```python
from build123d import *

# Parameters (mm, degrees)
SKETCH1_W               = 28.9
SKETCH1_H               = 5.8
BOSS_EXTRUDE1_DEPTH     = 2.5
CUT_EXTRUDE1_DEPTH      = 15.948662147
CUT_EXTRUDE1_DEPTH_BACK = 15.948662147
SKETCH2_R               = 0.525
FILL_START              = -2.5
FILL_PATTERN1_OUTLINE_R = 0.525
FILL_PATTERN1_DEPTH     = 5
SKETCH4_W               = 28.9
SKETCH4_H               = 0.2
BOSS_EXTRUDE2_DEPTH     = 2.5


# Read off the part's stored shape, not the designer's step: Fill Pattern1
with BuildPart() as part:
    # Sketch1 → Boss-Extrude1 (new, symmetric)
    with BuildSketch(Plane.XY):
        Rectangle(SKETCH1_W, SKETCH1_H)
    extrude(amount=BOSS_EXTRUDE1_DEPTH, both=True)

    # Sketch2 → Cut-Extrude1 (cut, two sides: drawn at the far end of the back side and taken through both)
    with BuildSketch(Plane.XY.offset(-CUT_EXTRUDE1_DEPTH_BACK)):
        Circle(SKETCH2_R)
    extrude(amount=CUT_EXTRUDE1_DEPTH + CUT_EXTRUDE1_DEPTH_BACK, mode=Mode.SUBTRACT)

    # Fill Pattern1 outline → Fill Pattern1 (cut)
    with BuildSketch(Plane.XY.offset(FILL_START)):
        with Locations((13.65, -1.125833025)):
            Circle(FILL_PATTERN1_OUTLINE_R)
        with Locations((-9.75, -1.125833025)):
            Circle(FILL_PATTERN1_OUTLINE_R)
        with Locations((-9.1, 0)):
            Circle(FILL_PATTERN1_OUTLINE_R)
        with Locations((-8.45, 1.125833025)):
            Circle(FILL_PATTERN1_OUTLINE_R)
        with Locations((-7.8, 2.25166605)):
            Circle(FILL_PATTERN1_OUTLINE_R)
        with Locations((-9.1, -2.25166605)):
            Circle(FILL_PATTERN1_OUTLINE_R)
        with Locations((-8.45, -1.125833025)):
            Circle(FILL_PATTERN1_OUTLINE_R)
        with Locations((-7.8, 0)):
            Circle(FILL_PATTERN1_OUTLINE_R)
        with Locations((-7.15, 1.125833025)):
            Circle(FILL_PATTERN1_OUTLINE_R)
        with Locations((-11.05, 1.125833025)):
            Circle(FILL_PATTERN1_OUTLINE_R)
        with Locations((-10.4, 2.25166605)):
            Circle(FILL_PATTERN1_OUTLINE_R)
        with Locations((-11.7, -2.25166605)):
            Circle(FILL_PATTERN1_OUTLINE_R)
        with Locations((-11.05, -1.125833025)):
            Circle(FILL_PATTERN1_OUTLINE_R)
        with Locations((-10.4, -2.25166605)):
            Circle(FILL_PATTERN1_OUTLINE_R)
        with Locations((-9.1, 2.25166605)):
            Circle(FILL_PATTERN1_OUTLINE_R)
        with Locations((-9.75, 1.125833025)):
            Circle(FILL_PATTERN1_OUTLINE_R)
        with Locations((-10.4, 0)):
            Circle(FILL_PATTERN1_OUTLINE_R)
        with Locations((-5.2, -2.25166605)):
            Circle(FILL_PATTERN1_OUTLINE_R)
        with Locations((-3.9, 2.25166605)):
            Circle(FILL_PATTERN1_OUTLINE_R)
        with Locations((-4.55, 1.125833025)):
            Circle(FILL_PATTERN1_OUTLINE_R)
        with Locations((-5.2, 0)):
            Circle(FILL_PATTERN1_OUTLINE_R)
        with Locations((-4.55, -1.125833025)):
            Circle(FILL_PATTERN1_OUTLINE_R)
        with Locations((-3.9, 0)):
            Circle(FILL_PATTERN1_OUTLINE_R)
        with Locations((-3.25, 1.125833025)):
            Circle(FILL_PATTERN1_OUTLINE_R)
        with Locations((-2.6, 2.25166605)):
            Circle(FILL_PATTERN1_OUTLINE_R)
        with Locations((-6.5, 0)):
            Circle(FILL_PATTERN1_OUTLINE_R)
        with Locations((-7.15, -1.125833025)):
            Circle(FILL_PATTERN1_OUTLINE_R)
        with Locations((-7.8, -2.25166605)):
            Circle(FILL_PATTERN1_OUTLINE_R)
        with Locations((-6.5, 2.25166605)):
            Circle(FILL_PATTERN1_OUTLINE_R)
        with Locations((-5.85, 1.125833025)):
            Circle(FILL_PATTERN1_OUTLINE_R)
        with Locations((-5.2, 2.25166605)):
            Circle(FILL_PATTERN1_OUTLINE_R)
        with Locations((-6.5, -2.25166605)):
            Circle(FILL_PATTERN1_OUTLINE_R)
        with Locations((-5.85, -1.125833025)):
            Circle(FILL_PATTERN1_OUTLINE_R)
        with Locations((-13.65, 1.125833025)):
            Circle(FILL_PATTERN1_OUTLINE_R)
        with Locations((-11.7, 2.25166605)):
            Circle(FILL_PATTERN1_OUTLINE_R)
        with Locations((-13, -2.25166605)):
            Circle(FILL_PATTERN1_OUTLINE_R)
        with Locations((-12.35, -1.125833025)):
            Circle(FILL_PATTERN1_OUTLINE_R)
        with Locations((-11.7, 0)):
            Circle(FILL_PATTERN1_OUTLINE_R)
        with Locations((-13, 2.25166605)):
            Circle(FILL_PATTERN1_OUTLINE_R)
        with Locations((-13.65, -1.125833025)):
            Circle(FILL_PATTERN1_OUTLINE_R)
        with Locations((-13, 0)):
            Circle(FILL_PATTERN1_OUTLINE_R)
        with Locations((-12.35, 1.125833025)):
            Circle(FILL_PATTERN1_OUTLINE_R)
        with Locations((7.15, -1.125833025)):
            Circle(FILL_PATTERN1_OUTLINE_R)
        with Locations((7.8, 0)):
            Circle(FILL_PATTERN1_OUTLINE_R)
        with Locations((8.45, 1.125833025)):
            Circle(FILL_PATTERN1_OUTLINE_R)
        with Locations((9.1, 2.25166605)):
            Circle(FILL_PATTERN1_OUTLINE_R)
        with Locations((7.8, -2.25166605)):
            Circle(FILL_PATTERN1_OUTLINE_R)
        with Locations((8.45, -1.125833025)):
            Circle(FILL_PATTERN1_OUTLINE_R)
        with Locations((9.1, 0)):
            Circle(FILL_PATTERN1_OUTLINE_R)
        with Locations((9.75, 1.125833025)):
            Circle(FILL_PATTERN1_OUTLINE_R)
        with Locations((5.85, 1.125833025)):
            Circle(FILL_PATTERN1_OUTLINE_R)
        with Locations((6.5, 2.25166605)):
            Circle(FILL_PATTERN1_OUTLINE_R)
        with Locations((5.2, -2.25166605)):
            Circle(FILL_PATTERN1_OUTLINE_R)
        with Locations((5.85, -1.125833025)):
            Circle(FILL_PATTERN1_OUTLINE_R)
        with Locations((6.5, -2.25166605)):
            Circle(FILL_PATTERN1_OUTLINE_R)
        with Locations((7.8, 2.25166605)):
            Circle(FILL_PATTERN1_OUTLINE_R)
        with Locations((7.15, 1.125833025)):
            Circle(FILL_PATTERN1_OUTLINE_R)
        with Locations((6.5, 0)):
            Circle(FILL_PATTERN1_OUTLINE_R)
        with Locations((11.7, -2.25166605)):
            Circle(FILL_PATTERN1_OUTLINE_R)
        with Locations((13, 2.25166605)):
            Circle(FILL_PATTERN1_OUTLINE_R)
        with Locations((12.35, 1.125833025)):
            Circle(FILL_PATTERN1_OUTLINE_R)
        with Locations((11.7, 0)):
            Circle(FILL_PATTERN1_OUTLINE_R)
        with Locations((13, -2.25166605)):
            Circle(FILL_PATTERN1_OUTLINE_R)
        with Locations((13.65, 1.125833025)):
            Circle(FILL_PATTERN1_OUTLINE_R)
        with Locations((13, 0)):
            Circle(FILL_PATTERN1_OUTLINE_R)
        with Locations((12.35, -1.125833025)):
            Circle(FILL_PATTERN1_OUTLINE_R)
        with Locations((10.4, 0)):
            Circle(FILL_PATTERN1_OUTLINE_R)
        with Locations((9.75, -1.125833025)):
            Circle(FILL_PATTERN1_OUTLINE_R)
        with Locations((9.1, -2.25166605)):
            Circle(FILL_PATTERN1_OUTLINE_R)
        with Locations((10.4, 2.25166605)):
            Circle(FILL_PATTERN1_OUTLINE_R)
        with Locations((11.05, 1.125833025)):
            Circle(FILL_PATTERN1_OUTLINE_R)
        with Locations((11.7, 2.25166605)):
            Circle(FILL_PATTERN1_OUTLINE_R)
        with Locations((10.4, -2.25166605)):
            Circle(FILL_PATTERN1_OUTLINE_R)
        with Locations((11.05, -1.125833025)):
            Circle(FILL_PATTERN1_OUTLINE_R)
        with Locations((-0.65, 1.125833025)):
            Circle(FILL_PATTERN1_OUTLINE_R)
        with Locations((0, 2.25166605)):
            Circle(FILL_PATTERN1_OUTLINE_R)
        with Locations((-1.3, -2.25166605)):
            Circle(FILL_PATTERN1_OUTLINE_R)
        with Locations((-0.65, -1.125833025)):
            Circle(FILL_PATTERN1_OUTLINE_R)
        with Locations((0.65, 1.125833025)):
            Circle(FILL_PATTERN1_OUTLINE_R)
        with Locations((1.3, 2.25166605)):
            Circle(FILL_PATTERN1_OUTLINE_R)
        with Locations((0, -2.25166605)):
            Circle(FILL_PATTERN1_OUTLINE_R)
        with Locations((0.65, -1.125833025)):
            Circle(FILL_PATTERN1_OUTLINE_R)
        with Locations((-3.9, -2.25166605)):
            Circle(FILL_PATTERN1_OUTLINE_R)
        with Locations((-3.25, -1.125833025)):
            Circle(FILL_PATTERN1_OUTLINE_R)
        with Locations((-2.6, 0)):
            Circle(FILL_PATTERN1_OUTLINE_R)
        with Locations((-1.95, 1.125833025)):
            Circle(FILL_PATTERN1_OUTLINE_R)
        with Locations((-1.3, 0)):
            Circle(FILL_PATTERN1_OUTLINE_R)
        with Locations((-1.95, -1.125833025)):
            Circle(FILL_PATTERN1_OUTLINE_R)
        with Locations((-2.6, -2.25166605)):
            Circle(FILL_PATTERN1_OUTLINE_R)
        with Locations((-1.3, 2.25166605)):
            Circle(FILL_PATTERN1_OUTLINE_R)
        with Locations((2.6, -2.25166605)):
            Circle(FILL_PATTERN1_OUTLINE_R)
        with Locations((3.25, -1.125833025)):
            Circle(FILL_PATTERN1_OUTLINE_R)
        with Locations((3.9, 0)):
            Circle(FILL_PATTERN1_OUTLINE_R)
        with Locations((4.55, 1.125833025)):
            Circle(FILL_PATTERN1_OUTLINE_R)
        with Locations((5.2, 0)):
            Circle(FILL_PATTERN1_OUTLINE_R)
        with Locations((4.55, -1.125833025)):
            Circle(FILL_PATTERN1_OUTLINE_R)
        with Locations((3.9, -2.25166605)):
            Circle(FILL_PATTERN1_OUTLINE_R)
        with Locations((5.2, 2.25166605)):
            Circle(FILL_PATTERN1_OUTLINE_R)
        with Locations((1.3, -2.25166605)):
            Circle(FILL_PATTERN1_OUTLINE_R)
        with Locations((2.6, 2.25166605)):
            Circle(FILL_PATTERN1_OUTLINE_R)
        with Locations((1.95, 1.125833025)):
            Circle(FILL_PATTERN1_OUTLINE_R)
        with Locations((1.3, 0)):
            Circle(FILL_PATTERN1_OUTLINE_R)
        with Locations((1.95, -1.125833025)):
            Circle(FILL_PATTERN1_OUTLINE_R)
        with Locations((2.6, 0)):
            Circle(FILL_PATTERN1_OUTLINE_R)
        with Locations((3.25, 1.125833025)):
            Circle(FILL_PATTERN1_OUTLINE_R)
        with Locations((3.9, 2.25166605)):
            Circle(FILL_PATTERN1_OUTLINE_R)
    extrude(amount=FILL_PATTERN1_DEPTH, mode=Mode.SUBTRACT)

    # Sketch4 → Boss-Extrude2 (add, symmetric)
    with BuildSketch(Plane.XY):
        with Locations((0, 3)):
            Rectangle(SKETCH4_W, SKETCH4_H)
        with Locations((0, -3)):
            Rectangle(SKETCH4_W, SKETCH4_H)
    extrude(amount=BOSS_EXTRUDE2_DEPTH, both=True)


solid = part.part
```
Part model, mm, in its own coordinate system. Round coordinates to 2 decimals unless told otherwise and drop trailing zeros. Answer in a Markdown table with one row per item. Add a question column.
Q1. Cut at A-A on y = -0.25. Give the number of separate pieces and of enclosed holes in the cut face, and give its area (3 significant figures).
Q2. Mould opens along X. For faces 1 (the face through (14.45, 0, 0)), 2 (the face through (3.483, -2.571, -0.035)) say: +X half, -X half, draft (parallel to the pull), parting line (faces both ways), or undercut.
Q3. Wall check: L1, parallel to Y at x = -10.4, z = 0.3 (3 decimals); L2, parallel to Y at x = -7.15, z = 1.05. Give the ranges that are in metal, low to high. Write a range as from..to.
Q4. Pin check, flat tips, straight feed: pin 1 (0.9 mm diameter, centred on x = -12.35, y = 1.13, fed in from -Z); pin 2 (1.4 mm diameter, centred on x = -10.4, y = 2.25, fed in from +Z). Stop position of each tip, or through.
Established:
| question | item | result |
|---|---|---|
| 1 | separate pieces | 22 |
| 1 | enclosed holes | 0 |
| 1 | area | 47.6 mm2 |
| 2 | face 1 | +X half |
| 2 | face 2 | undercut |
| 3 | L1 | y = -3.1..-2.777, -1.727..-0.525, 0.525..1.727, 2.777..3.1 |
| 3 | L2 | y = -3.1..-1.65, -0.6..0.6, 1.65..3.1 |
| 4 | pin 1 | passes through |
| 4 | pin 2 | stops at z = 2.5 |
